The model under review builds one solid part; all positions refer to its coordinate system, in mm. Coordinates: 2 decimals unless noted, no trailing zeros. Loops run counter-clockwise (first coordinate to the right, second up) from the corner with the lowest first, then second, coordinate; pieces in that order, holes last. Notation, with made-up numbers: M 34,14.5 L 80,14.5 A31 cw 80,44.5 Z; hole C -37,59.25 d6. An arc over 180 degrees is marked long. One line per item, written item: value.
```python
from build123d import *

# Parameters (mm, degrees)
F0_R     = 2.25
F1_DEPTH = 5


with BuildPart() as f1:
    # F0 (on Top) → F1 (new body)
    with BuildSketch(Plane.XY):
        Polygon((-155, -95), (155, -95), (155, 0), (135, 0), (135, 95), (-155, 95), align=None)
        with Locations((145, -80)):
            Circle(F0_R, mode=Mode.SUBTRACT)
        Polygon((87.5, -84), (84, -84), (-78.5, -84), (-78.5, -87.5), (-84, -87.5), (-84, -84), (-84, 78.5), (-87.5, 78.5), (-87.5, 84), (-84, 84), (78.5, 84), (78.5, 87.5), (84, 87.5), (84, 84), (84, -78.5), (87.5, -78.5), align=None, mode=Mode.SUBTRACT)
        with Locations((-145, 80)):
            Circle(F0_R, mode=Mode.SUBTRACT)
    extrude(amount=F1_DEPTH)


solid = f1.part
```
(1) Add section B-B on x = -12. State the section outline as (y, z) points.
Checks:
outline: M -95,0 L -84,0 L -84,5 L -95,5 Z; M 84,0 L 95,0 L 95,5 L 84,5 Z
(2) Insertion check: pin 1 Ø1.8 at (y, z) = (86, 3.5) entering from +X; pin 2 Ø6 at (x, y) = (-89.5, -51.5) entering from -Z; pin 3 Ø1.5 at (x, z) = (141, 2.5) entering from +Y. Each pin has a flat end and moves straight along its axis. Give the tip position at first contact, or say it passes through.
Checks:
pin 1: x = 135
pin 2: z = 0
pin 3: y = 0
(3) Add section C-C on z = 4.1. State the section outline as (x, y) points, then the cut area to 3 significant figures.
Checks:
outline: M -155,-95 L 155,-95 L 155,0 L 135,0 L 135,95 L -155,95 Z; hole C -145,80 d4.5; hole M -87.5,78.5 L -84,78.5 L -84,-87.5 L -78.5,-87.5 L -78.5,-84 L 87.5,-84 L 87.5,-78.5 L 84,-78.5 L 84,87.5 L 78.5,87.5 L 78.5,84 L -87.5,84 Z; hole C 145,-80 d4.5
area: 28,700 mm^2
(4) To check wall thickness, follow L1, parallel to X at y = -74.5, z = 0.65; L2, parallel to Y at x = 145, z = 3.2; L3, parallel to X at y = 33, z = 1.8. State the ranges of each line that lie inside material, in increasing order. Write a range as [from, to].
Checks:
L1: [-155, -84], [84, 155]
L2: [-95, -82.25], [-77.75, 0]
L3: [-155, -84], [84, 135]
(5) Add section A-A on y = -5. State the section outline as (x, z) points, then the cut area to 3 significant figures.
Checks:
outline: M -155,0 L -84,0 L -84,5 L -155,5 Z; M 84,0 L 155,0 L 155,5 L 84,5 Z
area: 710 mm^2
